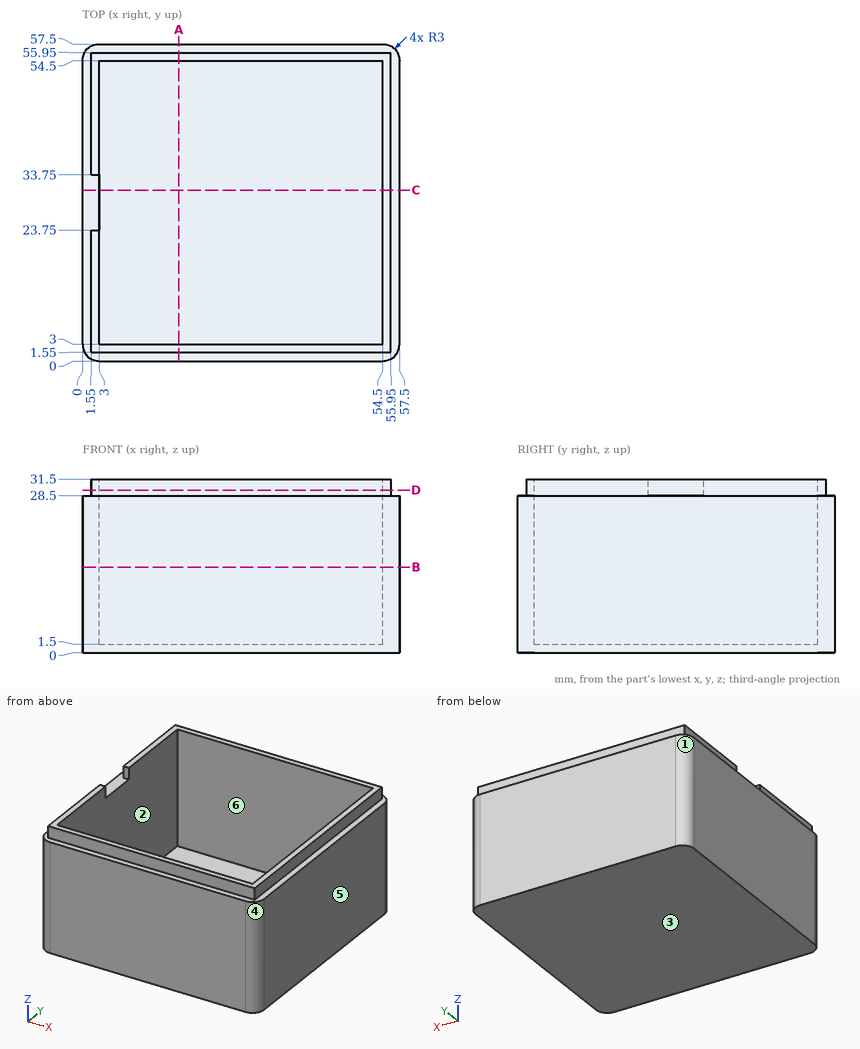
Source: three-view drawing plus pictorial views. Frame: mm from the lowest corner of the part. A direction names the side the tool comes from. Coordinates: 2 decimals unless noted, no trailing zeros. Order: outer loops, then holes, each group sorted by start corner. A loop starts at its lowest first (then second) coordinate and runs counter-clockwise, first axis right, second up.
Item 1: First-contact query: P1, Ø0.9, axis at y = 21, z = 30.5, coming from the +X side; P2, Ø5, axis at x = 18, y = 50.5, coming from the +Z side; P3, Ø3, axis at x = 36.5, z = 8.5, coming from the -Y side; P4, Ø1.5, axis at x = 34.5, z = 29.5, coming from the +Y side. Flat tips, straight axial feed; report the tip coordinate or a pass-through.
Output values:
P1: stops at x = 55.95
P2: stops at z = 1.5
P3: stops at y = 0
P4: stops at y = 55.95
Item 2: Set-up query: the marked faces 5 and 6. Return all of +Z, -Z, +X, -X, +Y, -Y with unobstructed straight access to the full face (end or side cutting, diameter ignored); none if empty.
Output values:
face 5: +Z, -Z, +X, +Y, -Y
face 6: +Z
Item 3: Cut plane D-D (z = 29.5). Return loops of the section in (x, y).
Output values:
outline: (1.55, 1.55) - (55.95, 1.55) - (55.95, 55.95) - (1.55, 55.95) - (1.55, 33.75) - (3, 33.75) - (3, 54.5) - (54.5, 54.5) - (54.5, 3) - (3, 3) - (3, 23.75) - (1.55, 23.75) - close
Item 4: Cut plane A-A (x = 17.5). Return loops of the section in (y, z), plus the area to 3 significant figures.
Output values:
outline: (0, 0) - (57.5, 0) - (57.5, 28.5) - (55.95, 28.5) - (55.95, 31.5) - (54.5, 31.5) - (54.5, 1.5) - (3, 1.5) - (3, 31.5) - (1.55, 31.5) - (1.55, 28.5) - (0, 28.5) - close
area: 257 mm2
Item 5: Pull-direction query (Y, two-part tool) for the marked faces 1, 2, 3 and 4; classes: pulls with the +Y half, pulls with the -Y half, needs draft (parallel to the pull), parting line crosses it, or undercut.
Output values:
face 1: pulls with the +Y half
face 2: undercut
face 3: needs draft
face 4: pulls with the -Y half
Item 6: Cut plane C-C (y = 31). Return loops of the section in (x, z), plus the area to 3 significant figures.
Output values:
outline: (0, 0) - (57.5, 0) - (57.5, 28.5) - (55.95, 28.5) - (55.95, 31.5) - (54.5, 31.5) - (54.5, 1.5) - (3, 1.5) - (3, 28.5) - (0, 28.5) - close
area: 253 mm2
Item 7: Cut plane B-B (z = 15.5). Return loops of the section in (x, y), plus the area to 3 significant figures.
Output values:
outline: (0, 3) arc R3 ccw to (3, 0) - (54.5, 0) arc R3 ccw to (57.5, 3) - (57.5, 54.5) arc R3 ccw to (54.5, 57.5) - (3, 57.5) arc R3 ccw to (0, 54.5) - close; hole (3, 3) - (54.5, 3) - (54.5, 54.5) - (3, 54.5) - close
area: 646 mm2
Item 8: Material intervals for line 1 (X direction, y = 22.5, z = 25.5); line 2 (X direction, y = 50, z = 30.5), sorted ascending.
Output values:
line 1: x = 0 to 3, 54.5 to 57.5
line 2: x = 1.55 to 3, 54.5 to 55.95
